Geometry: see drawing. Coordinates: mm, zero at the bounding-box minimum. Give positions to 0.01 mm unless a question says otherwise; leave off trailing zeros. Write each loop counter-clockwise with the first axis right and the second up, starting at its lowest first coordinate (ties: lowest second). Pieces come first, ordered by that corner, then holes. Notation, with made-up numbers: (10, -17) -> (48, -17) arc R10 cw to (48, -8) -> close; hole circle Ø1 at (7, 78). An arc over 180 degrees is marked (long way). Use CSV: the item, a comma, the result in double quotes. Start each with the question number.
1) Section D-D (y = 8.5). Output: boundary loops of the cut face in (x, z).
2) Material intervals for line 1 (Y direction, x = 6, z = 13); line 2 (Y direction, x = 10, z = 5); line 3 (X direction, y = 22, z = 13.75), sorted ascending. Write a range as [from, to].
3) Section C-C (x = 14). Output: boundary loops of the cut face in (y, z) (1 decimal).
4) Contact query for flat-ended pins moving along their axis: P1, Ø6, axis at y = 65.5, z = 4.5, coming from the -X side (1 decimal); P2, Ø1.5, axis at y = 71, z = 13, coming from the +X side (1 decimal); P3, Ø1.5, axis at y = 58.5, z = 19.5, coming from the -X side. Output: stop coordinate, or through.
5) Draft query along Y for the marked faces 1, 2, 3 and 4. Return one class per face: pulls with the +Y half, pulls with the -Y half, needs draft (parallel to the pull), parting line crosses it, or undercut.
6) Section A-A (x = 10.25). Output: boundary loops of the cut face in (y, z) (1 decimal).
7) Section B-B (z = 19.25). Output: boundary loops of the cut face in (x, y), plus the area to 3 significant figures.
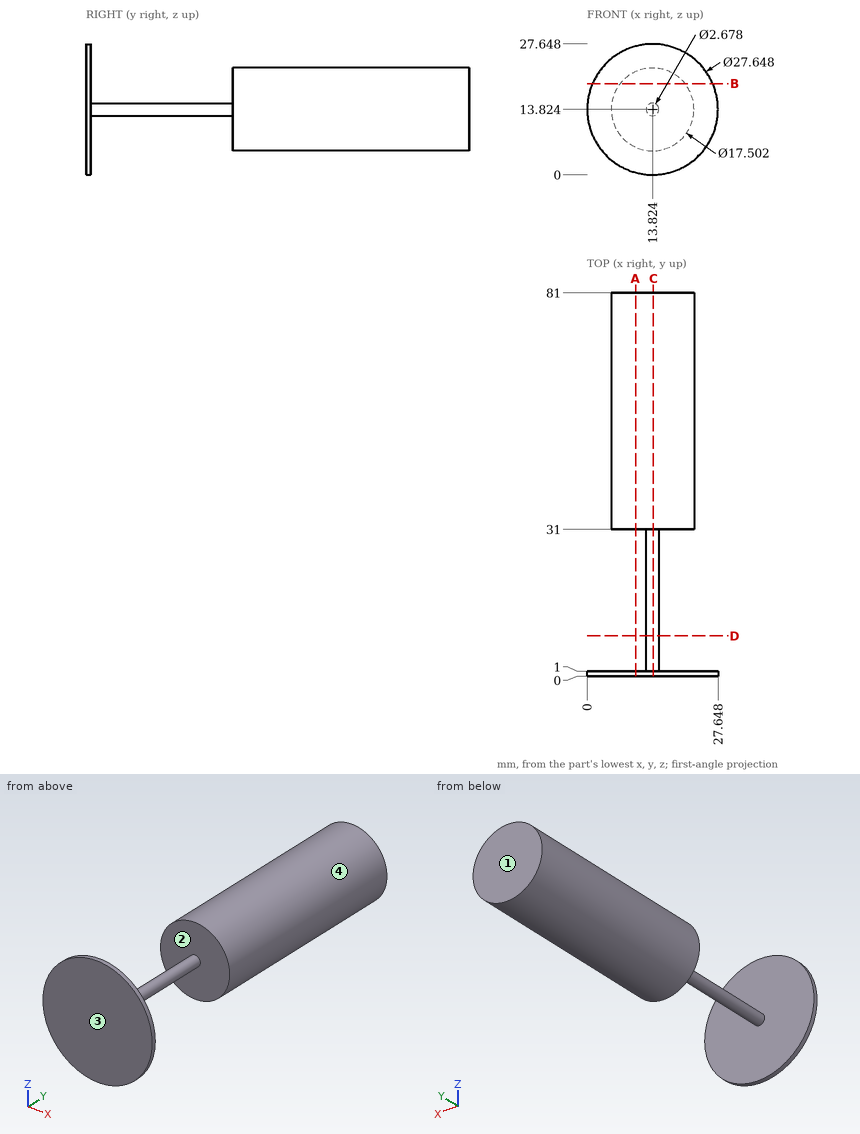
Answers follow:
1,outline,"circle Ø2.68 at (13.82, 13.82)"
2,line 1,"y = [0, 1], [31, 81]"
2,line 2,"y = [0, 1]"
2,line 3,"x = [12.49, 15.16]"
3,outline,"(0, 0) -> (1, 0) -> (1, 12.5) -> (31, 12.5) -> (31, 5.1) -> (81, 5.1) -> (81, 22.6) -> (31, 22.6) -> (31, 15.2) -> (1, 15.2) -> (1, 27.6) -> (0, 27.6) -> close"
4,P1,"stops at x = 7.8"
4,P2,"stops at x = 22.6"
4,P3,"stops at x = 6.59"
5,face 1,"pulls with the +Y half"
5,face 2,"undercut"
5,face 3,"pulls with the -Y half"
5,face 4,"needs draft"
6,outline,"(0, 0.5) -> (1, 0.5) -> (1, 27.2) -> (0, 27.2) -> close; (31, 5.8) -> (81, 5.8) -> (81, 21.8) -> (31, 21.8) -> close"
7,outline,"(1.11, 0) -> (26.54, 0) -> (26.54, 1) -> (1.11, 1) -> close; (6.96, 31) -> (20.69, 31) -> (20.69, 81) -> (6.96, 81) -> close"
7,area,"712 mm^2"
